Can you work these out from the model? Positions are in its coordinate system, mm. A direction names the side the tool comes from. Round coordinates to 2 decimals unless told otherwise and drop trailing zeros. Order: outer loops, then holes, each group sorted by start corner. A loop starts at its lowest first (then second) coordinate and runs counter-clockwise, first axis right, second up. Notation, with made-up numbers: M 24,15.5 L 67,15.5 A21 cw 67,43.5 Z; hole C -22,84 d5. An arc over 180 degrees is marked long. Answer as a JSON object with one key per item and string values. Group by question number.
```python
from build123d import *

# Parameters (mm, degrees)
SKETCH1_R           = 35
SKETCH1_R_2         = 25
BOSS_EXTRUDE1_DEPTH = 25
BOSS_EXTRUDE2_DEPTH = 60
FILLET2_R           = 10
FILLET3_R           = 5
FILLET4_R           = 2
SHELL1_T            = -1


with BuildPart() as part:
    # Sketch1 → Boss-Extrude1 (new body)
    # profile 1 of 2: a face of its own
    with BuildSketch(Plane(origin=(0, 0, 0), x_dir=(1, 0, 0), z_dir=(0, 1, 0))):
        with Locations(Location((-47.349258728, -4.926027286, 0), (0, 0, 270))):
            Circle(SKETCH1_R)
        with Locations((-47.349258728, -4.926027286)):
            Circle(SKETCH1_R_2, mode=Mode.SUBTRACT)
    # profile 2 of 2: a face of its own
    with BuildSketch(Plane(origin=(0, 0, 0), x_dir=(1, 0, 0), z_dir=(0, 1, 0))):
        with Locations((-47.349258728, -4.926027286)):
            Circle(SKETCH1_R_2)
    extrude(amount=BOSS_EXTRUDE1_DEPTH)

    # Sketch2 → Boss-Extrude2 (add)
    with BuildSketch(Plane(origin=(0, 25, 0), x_dir=(1, 0, 0), z_dir=(0, 1, 0))):
        with BuildLine():
            Line((-97.349258728, 55.073972714), (2.650741272, 55.073972714))
            ThreePointArc((2.650741272, 55.073972714), (9.721809084, 52.145040526), (12.650741272, 45.073972714))
            Line((12.650741272, 45.073972714), (12.650741272, -54.926027286))
            ThreePointArc((12.650741272, -54.926027286), (9.721809084, -61.997095098), (2.650741272, -64.926027286))
            Line((2.650741272, -64.926027286), (-97.349258728, -64.926027286))
            ThreePointArc((-97.349258728, -64.926027286), (-104.42032654, -61.997095098), (-107.349258728, -54.926027286))
            Line((-107.349258728, -54.926027286), (-107.349258728, 45.073972714))
            ThreePointArc((-107.349258728, 45.073972714), (-104.42032654, 52.145040526), (-97.349258728, 55.073972714))
        make_face()
    extrude(amount=BOSS_EXTRUDE2_DEPTH)

    # Fillet2
    fillet2_edges = [part.edges().sort_by_distance(p)[0] for p in [
        (-104.42032654, 25, -52.145040526),
        (-107.349258728, 25, 4.926027286),
        (-104.42032654, 25, 61.997095098),
        (-47.349258728, 25, 64.926027286),
        (9.721809084, 25, 61.997095098),
        (12.650741272, 25, 4.926027286),
        (9.721809084, 25, -52.145040526),
        (-47.349258728, 25, -55.073972714),
    ]]
    fillet(fillet2_edges, radius=FILLET2_R)

    # Fillet3
    fillet3_edges = [part.edges().sort_by_distance(p)[0] for p in [
        (-47.349258728, 25, -30.073972714),
    ]]
    fillet(fillet3_edges, radius=FILLET3_R)

    # Fillet4
    fillet4_edges = [part.edges().sort_by_distance(p)[0] for p in [
        (-47.349258728, 0, -30.073972714),
    ]]
    fillet(fillet4_edges, radius=FILLET4_R)

    # Shell1
    shell1_openings = [part.faces().sort_by_distance(p)[0] for p in [
        (-47.349258728, 85, 4.926027286),
    ]]
    offset(amount=SHELL1_T, openings=shell1_openings, kind=Kind.INTERSECTION)


solid = part.part
```
1) I need wall thicknesses on line 1 along Z through (x, y) = (-80, 51.5); line 2 along X through (y, z) = (77, 41); line 3 along X through (y, z) = (57.5, 55.5). Which ranges of each line are inside material? Lowest first, please.
2) If we section it at C-C on z = 52: Write out the boundary of the cut face in (x, y), plus the area to 3 significant figures.
3) For pin 1 (2 mm diameter, centred on x = -21, y = 18.5, fed in from +Z); pin 2 (1 mm diameter, centred on y = 28, z = 15, fed in from -X); pin 3 (4 mm diameter, centred on x = -67, z = -29, fed in from +Y), each with a flat end and sliding along its axis, tell me the tip position at first contact or that it passes through.
4) If we section it at D-D on y = 15: Write out the boundary of the cut face in (x, z), plus the area to 3 significant figures.
5) We'd pull the mould along Z, two halves only. Please class faces 1 (the face through (-103.783, 28.706, 4.226)), 2 (the face through (-46.649, 28.007, -52.222)), 3 (the face through (9.8, 59.65, 61.92)): +Z half, -Z half, draft (parallel to the pull), parting line (faces both ways), or undercut.
6) Which directions (+Z, -Z, +X, -X, +Y, -Y) give clear straight access to the entire face, cutting with the end or side of a thin tool? Please do faces 4 (the face through (8.94, 59.65, -51.51)), 5 (the face through (-68.646, 10.874, -22.849)), 6 (the face through (-48, 0, 4)).
7) If we section it at A-A on y = 48.5: Write out the boundary of the cut face in (x, z), plus the area to 3 significant figures.
8) If we section it at B-B on x = -1.5: Write out the boundary of the cut face in (y, z).
Findings:
{
 "1": {"line 1": "z = -55.07 to -54.07, 63.93 to 64.93", "line 2": "x = -107.35 to -106.35, 11.65 to 12.65", "line 3": "x = -107.33 to -106.33, 11.63 to 12.63"},
 "2": {"outline": "M -107.35,35 A10 ccw -97.35,25 L 2.65,25 A10 ccw 12.65,35 L 12.65,85 L 11.65,85 L 11.65,35 A9 cw 2.65,26 L -97.35,26 A9 cw -106.35,35 L -106.35,85 L -107.35,85 Z", "area": "230 mm^2"},
 "3": {"pin 1": "stops at z = 29.06", "pin 2": "stops at x = -104.95", "pin 3": "stops at y = 26"},
 "4": {"outline": "C -47.35,4.93 d70; hole C -47.35,4.93 d68", "area": "217 mm^2"},
 "5": {"face 1": "undercut", "face 2": "-Z half", "face 3": "+Z half"},
 "6": {"face 4": "+Y", "face 5": "-Y", "face 6": "+Z, -Z, +X, -X, -Y"},
 "7": {"outline": "M -107.35,-45.07 A10 ccw -97.35,-55.07 L 2.65,-55.07 A10 ccw 12.65,-45.07 L 12.65,54.93 A10 ccw 2.65,64.93 L -97.35,64.93 A10 ccw -107.35,54.93 Z; hole M -106.35,-45.07 A9 ccw -97.35,-54.07 L 2.65,-54.07 A9 ccw 11.65,-45.07 L 11.65,54.93 A9 ccw 2.65,63.93 L -97.35,63.93 A9 ccw -106.35,54.93 Z", "area": "460 mm^2"},
 "8": {"outline": "M 25,-45.07 A10 ccw 35,-55.07 L 85,-55.07 L 85,-54.07 L 35,-54.07 A9 cw 26,-45.07 L 26,54.93 A9 cw 35,63.93 L 85,63.93 L 85,64.93 L 35,64.93 A10 ccw 25,54.93 Z"}
}
